Here's the drawing with two shaded views (mm, measured from the low corner). I have some questions. Coordinates: 2 decimals unless noted, no trailing zeros. Write each loop counter-clockwise with the first axis right and the second up, starting at its lowest first coordinate (ties: lowest second). Pieces come first, ordered by that corner, then holes. Notation, with made-up numbers: (75.25, 5) -> (95.25, 5) arc R14 ccw to (95.25, 31) -> close; hole circle Ø1 at (-11.75, 76.25). An arc over 180 degrees is marked (long way). Use a Markdown table: item, result. Add a question column.
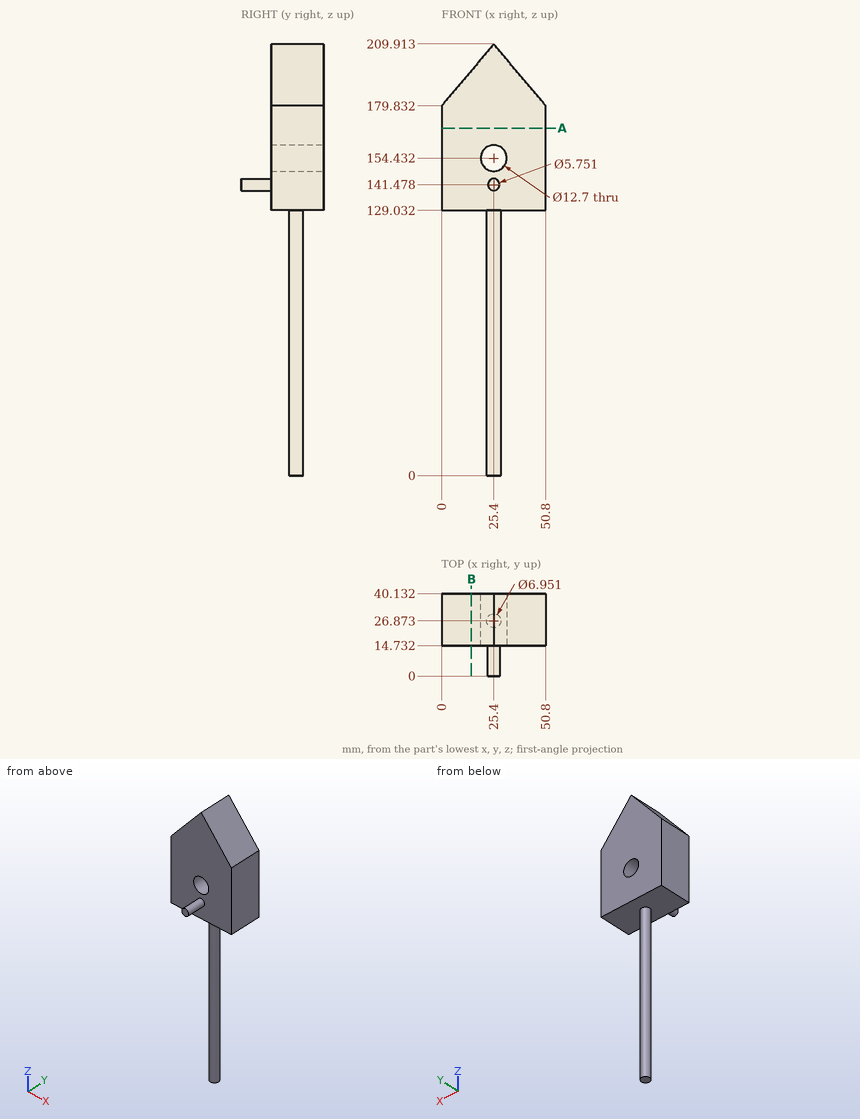
Q1. Suppose I cut it at A-A, the plane z = 169. Write out the boundary of the cut face in (x, y).
Q2. Suppose I cut it at B-B, the plane x = 14.5. Write out the boundary of the cut face in (y, z).
Q3. Please list where these lines run through material, in increasing order: line 1 (Z direction, x = 25.4, y = 29.5) (1 decimal); line 2 (Y direction, x = 21, z = 132); line 3 (Z direction, x = 31, y = 20) (1 decimal).
Q4. Will these pins go through, and if not, where does the flat tip stop? pin 1 (5 mm diameter, centred on y = 32, z = 35.5, fed in from +X) (1 decimal); pin 2 (10 mm diameter, centred on x = 22.5, z = 30, fed in from +Y); pin 3 (10 mm diameter, centred on x = 25.4, z = 154.432, fed in from +Y); pin 4 (6 mm diameter, centred on x = 7, y = 17, fed in from +Z) (1 decimal).
Answer key:
| question | item | result |
|---|---|---|
| 1 | outline | (0, 14.73) -> (50.8, 14.73) -> (50.8, 40.13) -> (0, 40.13) -> close |
| 2 | outline | (14.73, 129.03) -> (40.13, 129.03) -> (40.13, 197) -> (14.73, 197) -> close |
| 3 | line 1 | z = 0 to 148.1, 160.8 to 209.9 |
| 3 | line 2 | y = 14.73 to 40.13 |
| 3 | line 3 | z = 129 to 151.4, 157.4 to 203.3 |
| 4 | pin 1 | stops at x = 27.7 |
| 4 | pin 2 | stops at y = 30.35 |
| 4 | pin 3 | passes through |
| 4 | pin 4 | stops at z = 191.7 |
